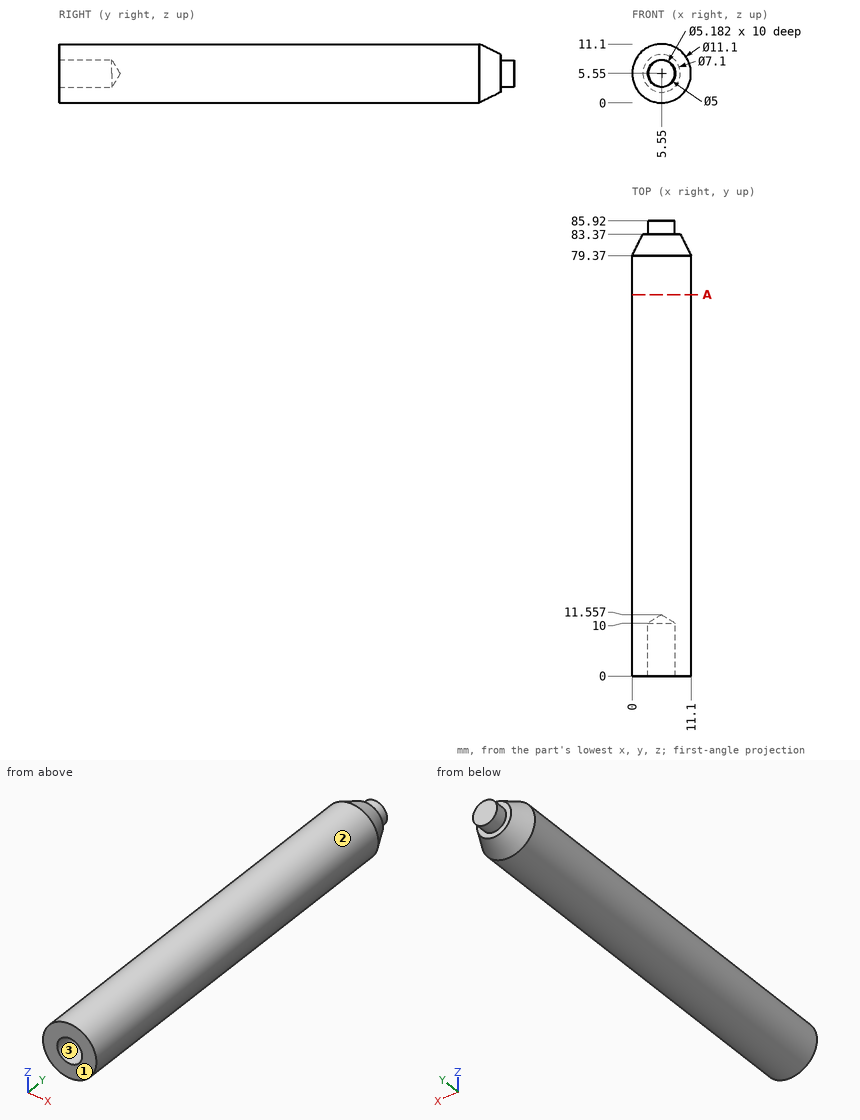
Can you work these out from the drawing? Everything is in mm from the part's minimum corner. Round coordinates to 2 decimals unless told otherwise and drop trailing zeros. Loops run counter-clockwise (first coordinate to the right, second up) from the corner with the lowest first, then second, coordinate; pieces in that order, holes last. Notation, with made-up numbers: (0.25, -22) - (53.25, -22) arc R14 ccw to (53.25, 2) - close; hole circle Ø3 at (62.5, -38.5). An arc over 180 degrees is marked (long way). Answer in a Markdown table with one row per item. Add a question column.
(1) I'm going to push flat-ended pins straight in: pin 1 (2 mm diameter, centred on y = 44.5, z = 5, fed in from +X); pin 2 (6 mm diameter, centred on x = 9.5, y = 68.5, fed in from -Z); pin 3 (4 mm diameter, centred on x = 5.55, z = 5.55, fed in from -Y) (1 decimal). Where does each tip first touch, or does it pass through?
(2) I need wall thicknesses on line 1 along Z through (x, y) = (5.55, 2.25); line 2 along Y through (x, z) = (8.5, 7.5). Which ranges of each line are inside material? Lowest first, please.
(3) If we mould it in two halves opening along Z, with no side actions, what happens to the marked faces 1, 2 and 3? For each: pulls with the +Z half, pulls with the -Z half, needs draft (parallel to the pull), parting line crosses it, or undercut.
(4) If we section it at A-A (y = 72): Please give me the cut outline in (x, z).
Model answer:
| question | item | result |
|---|---|---|
| 1 | pin 1 | stops at x = 11.1 |
| 1 | pin 2 | stops at z = 0.08 |
| 1 | pin 3 | stops at y = 10.4 |
| 2 | line 1 | z = 0 to 2.96, 8.14 to 11.1 |
| 2 | line 2 | y = 0 to 83.37 |
| 3 | face 1 | needs draft |
| 3 | face 2 | parting line crosses it |
| 3 | face 3 | undercut |
| 4 | outline | circle Ø11.1 at (5.55, 5.55) |
